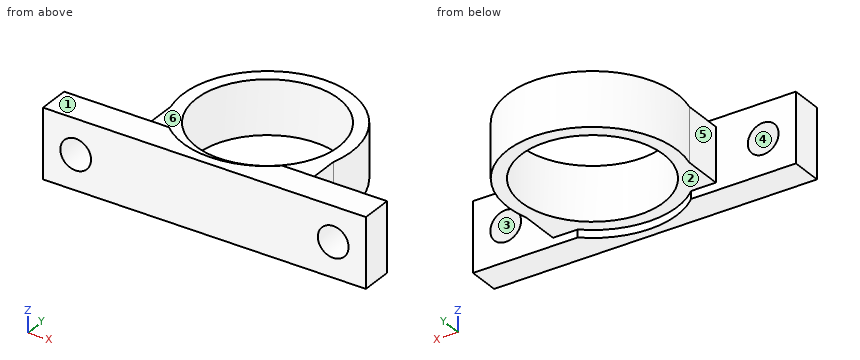
```python
from build123d import *

# Parameters (mm, degrees)
CROQUIS1_R              = 18.5
SALIENTE_EXTRUIR1_DEPTH = 18
CROQUIS2_R              = 17.5
CORTAR_EXTRUIR1_DEPTH   = 2
CROQUIS3_R              = 4
CORTAR_EXTRUIR2_DEPTH   = 9.2


with BuildPart() as part:
    # Croquis1 → Saliente-Extruir1 (new body)
    with BuildSketch(Plane.XY):
        with BuildLine():
            Line((0, 0), (-84, 0))
            Line((-84, 0), (-84, 8.2))
            Line((-84, 8.2), (-63.175317255, 8.2))
            Line((-63.175317255, 8.2), (-63.175317255, 18.532928764))
            ThreePointArc((-63.175317255, 18.532928764), (-42, 46.5), (-20.824682745, 18.532928764))
            Line((-20.824682745, 18.532928764), (-20.824682745, 8.2))
            Line((-20.824682745, 8.2), (0, 8.2))
            Line((0, 8.2), (0, 0))
        make_face()
        with Locations((-42, 24.5)):
            Circle(CROQUIS1_R, mode=Mode.SUBTRACT)
    extrude(amount=SALIENTE_EXTRUIR1_DEPTH)

    # Croquis2 → Cortar-Extruir1 (cut)
    with BuildSketch(Plane.XY.offset(18)):
        with BuildLine():
            Line((-20.824682745, 8.2), (-27.224682745, 8.2))
            ThreePointArc((-27.224682745, 8.2), (-42, 2.5), (-56.775317255, 8.2))
            Line((-56.775317255, 8.2), (-63.175317255, 8.2))
            Line((-63.175317255, 8.2), (-63.175317255, 18.532928764))
            ThreePointArc((-63.175317255, 18.532928764), (-42, 46.5), (-20.824682745, 18.532928764))
            Line((-20.824682745, 18.532928764), (-20.824682745, 8.2))
        make_face()
        with Locations((-42, 24.5)):
            Circle(CROQUIS2_R, mode=Mode.SUBTRACT)
    cortar_extruir1 = extrude(amount=-CORTAR_EXTRUIR1_DEPTH, mode=Mode.SUBTRACT)

    # Simetría1: Cortar-Extruir1 across plane
    add(cortar_extruir1.mirror(Plane.XY.offset(9)), mode=Mode.SUBTRACT)

    # Croquis3 → Cortar-Extruir2 (cut, through all)
    with BuildSketch(Plane(origin=(0, 8.2, 0), x_dir=(1, 0, 0), z_dir=(0, 1, 0))):
        with Locations((-8.5, -9)):
            Circle(CROQUIS3_R)
    cortar_extruir2 = extrude(amount=-CORTAR_EXTRUIR2_DEPTH, mode=Mode.SUBTRACT)

    # Simetría2: Cortar-Extruir2 across plane
    add(cortar_extruir2.mirror(Plane(origin=(-42, 0, 0), x_dir=(0, 0, 1), z_dir=(1, 0, 0))), mode=Mode.SUBTRACT)


solid = part.part
```
Geometry check sheet. Reference: the model listing, model coordinates, mm. Face numbers are marked on the shaded views. A direction names the side the tool comes from. Coordinates: 2 decimals unless noted, no trailing zeros. Order: outer loops, then holes, each group sorted by start corner. A loop starts at its lowest first (then second) coordinate and runs counter-clockwise, first axis right, second up. Notation, with made-up numbers: M 14.25,75 L 24.25,75 A27 ccw 24.25,108 Z; hole C 74,-19.75 d8. An arc over 180 degrees is marked long. Answer as a JSON object with one key per item and string values.
Q1. Cross-section at D-D on z = 3.75. Record the cut outline in (x, y), and give its area (3 significant figures).
Results are:
{"outline": "M -84,0 L 0,0 L 0,8.2 L -20.82,8.2 L -20.82,18.53 A22 ccw long -63.18,18.53 L -63.18,8.2 L -84,8.2 Z; hole C -42,24.5 d37", "area": "1,070 mm²"}
Q2. Cross-section at C-C on x = -75.5. Record the cut outline in (y, z).
Results are:
{"outline": "M 0,0 L 8.2,0 L 8.2,5 L 0,5 Z; M 0,13 L 8.2,13 L 8.2,18 L 0,18 Z"}
Q3. Scan lines: line 1 (X direction, y = 2.75, z = 9); line 2 (X direction, y = 24.5, z = 11); line 3 (Z direction, x = -75.5, y = 5.75). Record each from-to range of solid material in increasing order.
Results are:
{"line 1": "x = -84 to -79.5, -71.5 to -12.5, -4.5 to 0", "line 2": "x = -64 to -60.5, -23.5 to -20", "line 3": "z = 0 to 5, 13 to 18"}
Q4. Depth check by flat-ended pin: pin 1 Ø8 at (x, y) = (-27.5, 26) entering from +Z; pin 2 Ø1.5 at (y, z) = (16, 8) entering from -X; pin 3 Ø5 at (y, z) = (33, 8) entering from +X. Enter the tip coordinate at first touch or a pass-through.
Results are:
{"pin 1": "stops at z = 16", "pin 2": "stops at x = -63.18", "pin 3": "stops at x = -20.83"}
Q5. Cross-section at A-A on z = 9. Record the cut outline in (x, y), and give its area (3 significant figures).
Results are:
{"outline": "M -84,0 L -79.5,0 L -79.5,8.2 L -84,8.2 Z; M -71.5,0 L -12.5,0 L -12.5,8.2 L -20.82,8.2 L -20.82,18.53 A22 ccw long -63.18,18.53 L -63.18,8.2 L -71.5,8.2 Z; M -4.5,0 L 0,0 L 0,8.2 L -4.5,8.2 Z; hole C -42,24.5 d37", "area": "940 mm²"}
Q6. Cross-section at B-B on y = 24.5. Record the cut outline in (x, z), and give its area (3 significant figures).
Results are:
{"outline": "M -64,2 L -60.5,2 L -60.5,16 L -64,16 Z; M -23.5,2 L -20,2 L -20,16 L -23.5,16 Z", "area": "98.0 mm²"}
Q7. Release check for a two-part mould opening along Z. For the marked faces 1, 2 and 3 record: released by +Z, released by -Z, zero draft, split by the parting line, or undercut.
Results are:
{"face 1": "released by +Z", "face 2": "released by -Z", "face 3": "undercut"}
Q8. Tool access check on the marked faces 4, 5 and 6. Record the directions out of +Z, -Z, +X, -X, +Y, -Y that give a thin tool (end or side, any length) a straight path to the whole face; none if there is none.
Results are:
{"face 4": "+Y, -Y", "face 5": "+Z, -Z, -X", "face 6": "+Z, +Y"}
